Model file for the job. Use its own axes, mm. A direction names the side the tool comes from. Give positions to 0.01 mm unless a question says otherwise; leave off trailing zeros. Loops run counter-clockwise (first coordinate to the right, second up) from the corner with the lowest first, then second, coordinate; pieces in that order, holes last. Notation, with made-up numbers: (61, 69.5) - (110, 69.5) arc R10 ccw to (110, 74.5) - close; hole circle Ø11 at (77.25, 26.5). An arc over 180 degrees is marked (long way). Use a Markdown table: item, result.
from build123d import *

# Parameters (mm, degrees)
F1_DEPTH  = 35
F3_W      = 14.1933254312
F3_H      = 10
F4_DEPTH  = 5
F6_DEPTH  = 5
F8_DEPTH  = 0.5
F9_DEPTH  = 200
F10_DEPTH = 1.71
F11_DEPTH = 4


with BuildPart() as f1:
    # F0 (on Right) → F1 (new body, symmetric)
    with BuildSketch(Plane.YZ):
        Polygon((4.0779394949, -1.9816074769), (-5.5346774645, 0.7747660812), (-3.7443463919, 7.0183925231), (-6.5346774645, 7.0183925231), (-6.5346774645, -2.9816074769), (7.6586479667, -2.9816074769), (7.6586479667, 7.0183925231), (6.6586479667, 7.0183925231), align=None)
    extrude(amount=F1_DEPTH, both=True)


with BuildPart() as f1_1:
    # F2: moved
    add(f1.part.moved(Location((0, 0, 2.9817))))

    # F3 (on face) → F4 (join)
    with BuildSketch(Plane(origin=(-35, 0, 0), x_dir=(0, -1, 0), z_dir=(-1, 0, 0))):
        with Locations((-0.5619852511, 5.0000925231)):
            Rectangle(F3_W, F3_H)
    extrude(amount=F4_DEPTH)

    # F5 (on face) → F6 (join)
    with BuildSketch(Plane.YZ.offset(35)):
        Polygon((-3.7443463919, 10.0000925231), (-6.5346774645, 10.0000925231), (-6.5346774645, 9.25231e-05), (7.6586479667, 9.25231e-05), (7.6586479667, 10.0000925231), (6.6586479667, 10.0000925231), (4.0779394949, 1.0000925231), (-5.5346774645, 3.7564660812), align=None)
        Polygon((6.6586479667, 10.0000925231), (-3.7443463919, 10.0000925231), (-5.5346774645, 3.7564660812), (4.0779394949, 1.0000925231), align=None)
    extrude(amount=F6_DEPTH)

    # F8 (add): a face of the model
    f8_faces = [f1_1.faces().sort_by_distance(p)[0] for p in [
        (0, -6.5346774645, 5.0000925231),
    ]]
    extrude(f8_faces, amount=F8_DEPTH)

    # F7 (on face) → F9 (cut)
    with BuildSketch(Plane(origin=(0, 0.574809482, 2.00459889), x_dir=(1, 0, 0), z_dir=(0, 0.2756373558, 0.9612616959))):
        Polygon((15, 3.6443041761), (0, 3.6443041761), (-15, 3.6443041761), (-15, -6.3556958239), (15, -6.3556958239), align=None)
    extrude(amount=-F9_DEPTH, mode=Mode.SUBTRACT)

    # F10 (add): a face of the model
    f10_faces = [f1_1.faces().sort_by_distance(p)[0] for p in [
        (0, -7.0346774645, 5.0000925231),
    ]]
    extrude(f10_faces, amount=F10_DEPTH)

    # F11 (add): a face of the model
    f11_faces = [f1_1.faces().sort_by_distance(p)[0] for p in [
        (0, 7.6586479667, 5.0000925231),
    ]]
    extrude(f11_faces, amount=F11_DEPTH)


solid = f1_1.part
(1) 3-axis set-ups, long thin cutter, end or side, ignore diameter. For faces 1 (the flat face through (1, -5, 10)), 2 (the flat face through (25.14, -0.66, 2.36)): which of +Z, -Z, +X, -X, +Y, -Y reach the whole face in a straight line?
Computed:
| item | result |
|---|---|
| face 1 | +Z, +X, -X, +Y, -Y |
| face 2 | none |
(2) Slice it at B-B, the plane z = 8. Write the cut outline in (x, y), plus the area to 3 significant figures.
Computed:
| item | result |
|---|---|
| outline | (-40, -8.74) - (40, -8.74) - (40, 11.66) - (-40, 11.66) - close; hole (-35, -4.32) - (35, -4.32) - (35, 6.09) - (-35, 6.09) - close |
| area | 904 mm² |
(3) Slice it at C-C, the plane y = -4.5. Write the cut outline in (x, z).
Computed:
| item | result |
|---|---|
| outline | (-40, 0) - (-15, 0) - (-15, 3.46) - (-35, 3.46) - (-35, 7.36) - (35, 7.36) - (35, 3.46) - (15, 3.46) - (15, 0) - (40, 0) - (40, 10) - (-40, 10) - close |
(4) Mould opens along X. For faces 3 (the flat face through (-15, -2, 1)), 4 (the flat face through (-1, -8.745, 5)), 5 (the flat face through (-40, 1, 5)) say: pulls with the +X half, pulls with the -X half, needs draft (parallel to the pull), parting line crosses it, or undercut.
Computed:
| item | result |
|---|---|
| face 3 | undercut |
| face 4 | needs draft |
| face 5 | pulls with the -X half |
(5) Slice it at A-A, the plane x = 1. Write the cut outline in (y, z).
Computed:
| item | result |
|---|---|
| outline | (-8.74, 0) - (-6.61, 0) - (-3.74, 10) - (-8.74, 10) - close; (3.79, 0) - (11.66, 0) - (11.66, 10) - (6.66, 10) - close |
(6) Slice it at D-D, the plane x = 32. Write the cut outline in (y, z).
Computed:
| item | result |
|---|---|
| outline | (-8.74, 0) - (11.66, 0) - (11.66, 10) - (6.66, 10) - (4.08, 1) - (-5.53, 3.76) - (-3.74, 10) - (-8.74, 10) - close |
(7) Drill centre lines: probe 1 along X at (y, z) = (-2.5, 7.75); probe 2 along Y at (x, z) = (-6.5, 1.25); probe 3 along Y at (x, z) = (9, 9.75). Where is each one in solid material? Low to high. Write a range as [from, to].
Computed:
| item | result |
|---|---|
| probe 1 | [-40, -35], [35, 40] |
| probe 2 | [-8.74, -6.25], [4.15, 11.66] |
| probe 3 | [-8.74, -3.82], [6.59, 11.66] |
